Verification items for the finished model (mm, model axes). Face numbers are marked on the shaded views. A direction names the side the tool comes from. Round coordinates to 2 decimals unless told otherwise and drop trailing zeros. Write each loop counter-clockwise with the first axis right and the second up, starting at its lowest first coordinate (ties: lowest second). Pieces come first, ordered by that corner, then holes. Notation, with made-up numbers: M 0,-15 L 58,-15 A34 cw 58,24 Z; hole C 53,28.5 d1. An arc over 180 degrees is marked long. One line per question, with ' | ' between items.
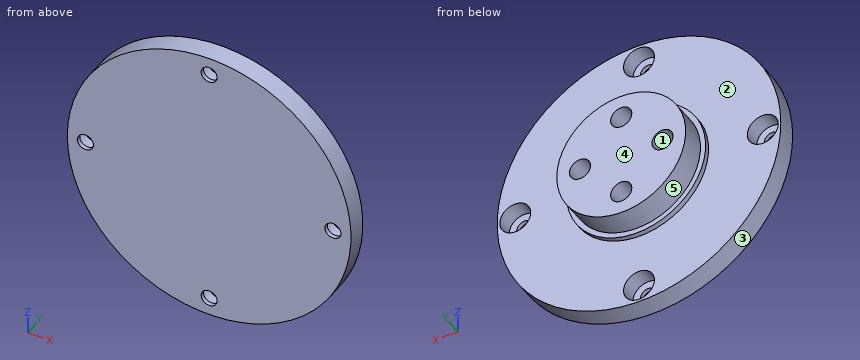
Autodesk Inventor part; units mm, degrees
ref_plane "YZ Plane" through (0, 0, 0) normal (1, 0, 0) x (0, 1, 0)
ref_plane "XZ Plane" through (0, 0, 0) normal (0, 1, 0) x (-1, 0, 0)
ref_plane "XY Plane" through (0, 0, 0) normal (0, 0, 1) x (1, 0, 0)
sketch "Szkic1" plane through (0, 0, 0) normal (0, 1, 0) x (-1, 0, 0)
  circle A0 centre (0, 0) radius 27.5
  dimension "d0" = 55
extrude "Wyciągnięcie proste1" add sketch "Szkic1" along normal blind 4
sketch "Szkic2" plane through (0, 4, 0) normal (0, 1, 0) x (1, 0, 0)
  circle A0 centre (-24, 0) radius 1.55
  circle A1 centre (0, -24) radius 1.55
  circle A2 centre (24, 0) radius 1.55
  circle A3 centre (0, 24) radius 1.55
  point P0 (0, 0)
  dimension "d3" = 3.1
  dimension "d4" = 24
  dimension "d7" = 360
extrude "Wyciągnięcie proste2" cut sketch "Szkic2" against normal up to surface (4 mm away)
sketch "Szkic3" plane through (0, 4, 0) normal (0, 1, 0) x (1, 0, 0)
  circle A0 centre (0, 0) radius 12.5
  dimension "d11" = 25
extrude "Wyciągnięcie proste3" add sketch "Szkic3" along normal blind 6
sketch "Szkic4" plane through (0, 10, 0) normal (0, 1, 0) x (1, 0, 0)
  circle A0 centre (-8, 0) radius 2.05
  circle A1 centre (0, -8) radius 2.05
  circle A2 centre (8, 0) radius 2.05
  circle A3 centre (0, 8) radius 2.05
  point P0 (0, 0)
  dimension "d14" = 4.1
  dimension "d17" = 360
  dimension "d19" = 8
extrude "Wyciągnięcie proste4" cut sketch "Szkic4" against normal blind 8
sketch "Szkic5" plane through (0, 4, 0) normal (0, 1, 0) x (1, 0, 0)
  circle A0 centre (-24, 0) radius 1.55
  circle A1 centre (-24, 0) radius 3
  circle A2 centre (0, -24) radius 3
  circle A3 centre (24, 0) radius 3
  circle A4 centre (0, 24) radius 3
  point P0 (0, 0)
  dimension "d22" = 6
  dimension "d27" = 360
extrude "Wyciągnięcie proste5" cut sketch "Szkic5" against normal blind 3.2
sketch "Szkic6" plane through (0, 4, 0) normal (0, 1, 0) x (1, 0, 0)
  circle A0 centre (0, 0) radius 13.5
  dimension "d29" = 27
extrude "Wyciągnięcie proste6" add sketch "Szkic6" along normal blind 1
properties part number "_Drukowanie 3D"
1. Mould release check, pull along X, two halves, no side actions. Record for the marked faces 1, 2 and 3: pulls with the +X half, pulls with the -X half, needs draft (parallel to the pull), parting line crosses it, or undercut.
Results:
face 1: undercut | face 2: needs draft | face 3: parting line crosses it
2. Tool access check on the marked faces 4 and 5. Record the directions out of +Z, -Z, +X, -X, +Y, -Y that give a thin tool (end or side, any length) a straight path to the whole face; none if there is none.
Results:
face 4: +Z, -Z, +X, -X, +Y | face 5: +Y
3. Section check A-A, the plane z = 0. Count the separate pieces of the cut face and the enclosed holes in it, then the cut area to 3 significant figures.
Results:
separate pieces: 3 | enclosed holes: 2 | area: 271 mm2
4. Go/stop test with flat-tipped pins: P1, Ø3, axis at x = -1, z = -25, coming from the +Y side; P2, Ø3.5, axis at x = 8, z = 0, coming from the +Y side; P3, Ø9.5, axis at x = 0, z = -24, coming from the +Y side. Record where each tip stops, or that it passes through.
Results:
P1: stops at y = 0.8 | P2: stops at y = 5 | P3: stops at y = 4
5. Section check B-B, the plane x = -8. Record the cut outline in (y, z), then the cut area to 3 significant figures.
Results:
outline: M 0,-26.31 L 4,-26.31 L 4,-10.87 L 5,-10.87 L 5,-9.6 L 10,-9.6 L 10,-2.05 L 5,-2.05 L 5,2.05 L 10,2.05 L 10,9.6 L 5,9.6 L 5,10.87 L 4,10.87 L 4,26.31 L 0,26.31 Z; hole M 2,-2.05 L 4,-2.05 L 4,2.05 L 2,2.05 Z | area: 300 mm2
6. Section check C-C, the plane y = 8. Record the cut outline in (x, z), then the cut area to 3 significant figures.
Results:
outline: C 0,0 d25; hole C -8,0 d4.1; hole C 0,-8 d4.1; hole C 0,8 d4.1; hole C 8,0 d4.1 | area: 438 mm2
7. Thickness scan on line 1 (Z direction, x = 0, y = 7.2); line 2 (Z direction, x = 0, y = 3.15). Record the ranges inside material, lowest first.
Results:
line 1: z = -12.5 to -10.05, -5.95 to 5.95, 10.05 to 12.5 | line 2: z = -27.5 to -27, -21 to -10.05, -5.95 to 5.95, 10.05 to 21, 27 to 27.5
